```python
from build123d import *

# Parameters (mm, degrees)
ESQUISSE1_R                  = 7.8
BOSS_EXTRU_1_DEPTH           = 2.675
BOSS_EXTRU_1_TAPER           = 30
BOSS_EXTRU_1_OTHER_WAY_DEPTH = 2.675
BOSS_EXTRU_1_OTHER_WAY_TAPER = 30
BOSS_EXTRU_2_DEPTH           = 0.19
BOSS_EXTRU_2_DEPTH_BACK      = 0.19
ENL_V_MAT_EXTRU_1_DEPTH      = 1.19
ESQUISSE4_R                  = 0.604402157
ENL_V_MAT_EXTRU_2_DEPTH      = 0.2
ESQUISSE5_W                  = 1.06783848
ESQUISSE5_H                  = 1.016251764
ENL_V_MAT_EXTRU_3_DEPTH      = 0.2
CONG_1_R                     = 0.5


with BuildPart() as part:
    # Esquisse1 → Boss.-Extru.1 (new body)
    with BuildSketch(Plane(origin=(0, 0, 0), x_dir=(1, 0, 0), z_dir=(0, 1, 0))):
        Circle(ESQUISSE1_R)
    extrude(amount=BOSS_EXTRU_1_DEPTH, taper=BOSS_EXTRU_1_TAPER)

    # Esquisse1 → Boss.-Extru.1 other way (add)
    with BuildSketch(Plane(origin=(0, 0, 0), x_dir=(1, 0, 0), z_dir=(0, 1, 0))):
        Circle(ESQUISSE1_R)
    extrude(amount=-BOSS_EXTRU_1_OTHER_WAY_DEPTH, taper=BOSS_EXTRU_1_OTHER_WAY_TAPER)

    # Esquisse2 → Boss.-Extru.2 (add, two sides: drawn at the far end of the back side and taken through both)
    with BuildSketch(Plane(origin=(0, 0, 0), x_dir=(1, 0, 0), z_dir=(0, 1, 0)).offset(-BOSS_EXTRU_2_DEPTH_BACK)):
        with BuildLine():
            Line((1.969010028, -12), (1.969010028, -5.174670877))
            Line((1.969010028, -5.174670877), (0.570530435, -5.174670877))
            Line((0.570530435, -5.174670877), (0.570530435, -12))
            Line((0.570530435, -12), (1.014706926, -12))
            Line((1.014706926, -12), (1.014706926, -18.3))
            ThreePointArc((1.014706926, -18.3), (1.271696248, -18.556989322), (1.52868557, -18.3))
            Line((1.52868557, -18.3), (1.52868557, -12))
            Line((1.52868557, -12), (1.969010028, -12))
        make_face()
        with BuildLine():
            Line((4.069208585, -18.3), (4.069208585, -12))
            Line((4.069208585, -12), (4.512824501, -12))
            Line((4.512824501, -12), (4.512824501, -5.174670877))
            Line((4.512824501, -5.174670877), (3.110830289, -5.174670877))
            Line((3.110830289, -5.174670877), (3.110830289, -12))
            Line((3.110830289, -12), (3.555229941, -12))
            Line((3.555229941, -12), (3.555229941, -18.3))
            ThreePointArc((3.555229941, -18.3), (3.812219263, -18.556989322), (4.069208585, -18.3))
        make_face()
        with BuildLine():
            Line((-0.570530435, -5.174670877), (-0.570530435, -12))
            Line((-0.570530435, -12), (-1.014706926, -12))
            Line((-1.014706926, -12), (-1.014706926, -18.3))
            ThreePointArc((-1.014706926, -18.3), (-1.271696248, -18.556989322), (-1.52868557, -18.3))
            Line((-1.52868557, -18.3), (-1.52868557, -12))
            Line((-1.52868557, -12), (-1.969010028, -12))
            Line((-1.969010028, -12), (-1.969010028, -5.174670877))
            Line((-1.969010028, -5.174670877), (-0.570530435, -5.174670877))
        make_face()
        with BuildLine():
            Line((-4.512824501, -5.174670877), (-3.110830289, -5.174670877))
            Line((-3.110830289, -5.174670877), (-3.110830289, -12))
            Line((-3.110830289, -12), (-3.555229941, -12))
            Line((-3.555229941, -12), (-3.555229941, -18.3))
            ThreePointArc((-3.555229941, -18.3), (-3.812219263, -18.556989322), (-4.069208585, -18.3))
            Line((-4.069208585, -18.3), (-4.069208585, -12))
            Line((-4.069208585, -12), (-4.512824501, -12))
            Line((-4.512824501, -12), (-4.512824501, -5.174670877))
        make_face()
    extrude(amount=BOSS_EXTRU_2_DEPTH + BOSS_EXTRU_2_DEPTH_BACK)

    # Esquisse3 → Enlèv. mat.-Extru.1 (cut)
    with BuildSketch(Plane(origin=(0, 0.19, 0), x_dir=(1, 0, 0), z_dir=(0, 1, 0))):
        with BuildLine():
            Line((-4.512824501, -10.241819979), (-4.512824501, -11.117491511))
            ThreePointArc((-4.512824501, -11.117491511), (-4.074988736, -10.679655745), (-4.512824501, -10.241819979))
        make_face()
    extrude(amount=-ENL_V_MAT_EXTRU_1_DEPTH, mode=Mode.SUBTRACT)

    # Esquisse4 → Enlèv. mat.-Extru.2 (cut)
    with BuildSketch(Plane(origin=(0, 2.675, 0), x_dir=(1, 0, 0), z_dir=(0, 1, 0))):
        with Locations(Location((0, 0, 0), (0, 0, 270))):
            Circle(ESQUISSE4_R)
    extrude(amount=-ENL_V_MAT_EXTRU_2_DEPTH, mode=Mode.SUBTRACT)

    # Esquisse5 → Enlèv. mat.-Extru.3 (cut)
    with BuildSketch(Plane.XZ.offset(2.675)):
        Rectangle(ESQUISSE5_W, ESQUISSE5_H)
    extrude(amount=-ENL_V_MAT_EXTRU_3_DEPTH, mode=Mode.SUBTRACT)

    # Congé1
    cong_1_edges = [part.edges().sort_by_distance(p)[0] for p in [
        (-6.25558803, 2.675, 0),
    ]]
    fillet(cong_1_edges, radius=CONG_1_R)


solid = part.part
```
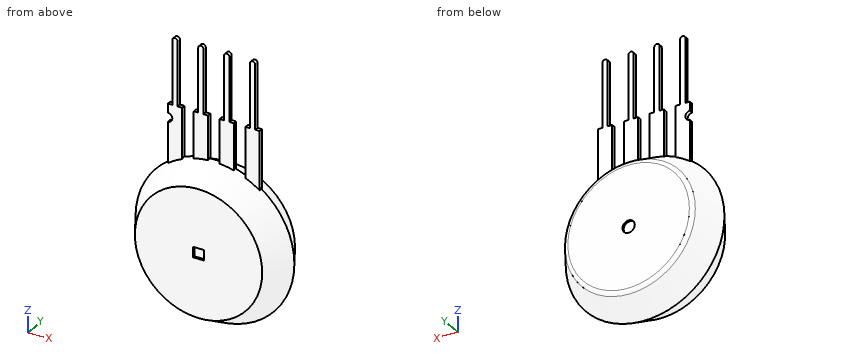
Could you check a few things on this model? Use its own coordinates, in mm. Coordinates: 2 decimals unless noted, no trailing zeros. Loops run counter-clockwise (first coordinate to the right, second up) from the corner with the lowest first, then second, coordinate; pieces in that order, holes last.
1) Please list where these lines run through material, in increasing order: line 1 along Y through (x, z) = (4, 17); line 2 along Y through (x, z) = (0, 0) (3 decimals); line 3 along X through (y, z) = (-0.9, 3.25).
Reported:
line 1: y = -0.19 to 0.19
line 2: y = -2.475 to 2.475
line 3: x = -6.51 to 6.51
2) Imagine slicing it at A-A (z = 16.75). List the corners of the cut face in (x, y) for me, and give its area (3 significant figures).
Reported:
outline: (-4.07, -0.19) - (-3.56, -0.19) - (-3.56, 0.19) - (-4.07, 0.19) - close; (-1.53, -0.19) - (-1.01, -0.19) - (-1.01, 0.19) - (-1.53, 0.19) - close; (1.01, -0.19) - (1.53, -0.19) - (1.53, 0.19) - (1.01, 0.19) - close; (3.56, -0.19) - (4.07, -0.19) - (4.07, 0.19) - (3.56, 0.19) - close
area: 0.781 mm2
3) Imagine slicing it at D-D (y = -1.1). List the corners of the cut face in (x, z) for me.
Reported:
outline: circle Ø14.33 at (0, 0)
4) Imagine slicing it at B-B (x = 0). List the corners of the cut face in (y, z) for me (3 decimals), and give its area (3 significant figures).
Reported:
outline: (-2.675, -6.256) - (0, -7.8) - (2.425, -6.4) arc R0.5 ccw to (2.675, -5.967) - (2.675, -0.604) - (2.475, -0.604) - (2.475, 0.604) - (2.675, 0.604) - (2.675, 5.967) arc R0.5 ccw to (2.425, 6.4) - (0, 7.8) - (-2.675, 6.256) - (-2.675, 0.508) - (-2.475, 0.508) - (-2.475, -0.508) - (-2.675, -0.508) - close
area: 74.7 mm2
5) Imagine slicing it at C-C (z = 9.5). List the corners of the cut face in (x, y) for me, and give its area (3 significant figures).
Reported:
outline: (-4.51, -0.19) - (-3.11, -0.19) - (-3.11, 0.19) - (-4.51, 0.19) - close; (-1.97, -0.19) - (-0.57, -0.19) - (-0.57, 0.19) - (-1.97, 0.19) - close; (0.57, -0.19) - (1.97, -0.19) - (1.97, 0.19) - (0.57, 0.19) - close; (3.11, -0.19) - (4.51, -0.19) - (4.51, 0.19) - (3.11, 0.19) - close
area: 2.13 mm2
6) Will these pins go through, and if not, where does the flat tip stop? pin 1 Ø0.7 at (x, z) = (3.5, 15) entering from -Y; pin 2 Ø0.7 at (x, z) = (1.5, 13.5) entering from +Y; pin 3 Ø1 at (x, y) = (1, -0.5) entering from -Z.
Reported:
pin 1: stops at y = -0.19
pin 2: stops at y = 0.19
pin 3: stops at z = -7.74
